Source: CAD feature listing. Evaluate the final solid. Frame: model axes, mm. A direction names the side the tool comes from. Coordinates: 2 decimals unless noted, no trailing zeros. Loops run counter-clockwise (first coordinate to the right, second up) from the corner with the lowest first, then second, coordinate; pieces in that order, holes last.
```python
from build123d import *

# Parameters (mm, degrees)
SKETCH_1_W          = 34
SKETCH_1_H          = 10
EXTRUDE_1_DEPTH     = 2
FILLET_1_R          = 3
SKETCH_2_R          = 1.5
CUT_EXTRUDE_1_DEPTH = 2
EXTRUDE_2_DEPTH     = 11
SKETCH_5_W          = 21
SKETCH_5_H          = 14
EXTRUDE_4_DEPTH     = 2
EXTRUDE_4_TAPER     = 48
SKETCH_6_W          = 15
SKETCH_6_H          = 8
CUT_EXTRUDE_2_DEPTH = 0.3
EXTRUDE_5_DEPTH     = 8


with BuildPart() as part:
    # 草图1 → 凸台-拉伸1 (new body)
    with BuildSketch(Plane.XY):
        Rectangle(SKETCH_1_W, SKETCH_1_H)
    extrude(amount=EXTRUDE_1_DEPTH)

    # 圆角1
    fillet_1_edges = [part.edges().sort_by_distance(p)[0] for p in [
        (-17, 5, 1),
        (17, 5, 1),
        (17, -5, 1),
        (-17, -5, 1),
    ]]
    fillet(fillet_1_edges, radius=FILLET_1_R)

    # 草图2 → 切除-拉伸1 (cut)
    with BuildSketch(Plane.XY.offset(2)):
        with Locations((-14, 0)):
            Circle(SKETCH_2_R)
        with Locations(Location((14, 0, 0), (0, 0, 180))):
            Circle(SKETCH_2_R)
    extrude(amount=-CUT_EXTRUDE_1_DEPTH, mode=Mode.SUBTRACT)

    # 草图3 → 凸台-拉伸2 (add)
    with BuildSketch(Plane.XY.offset(2)):
        with BuildLine():
            Line((12, -5), (-12, -5))
            Line((-12, -5), (-12, -4))
            Line((-12, -4), (-7.5, -4))
            ThreePointArc((-7.5, -4), (-5, -1.5), (-7.5, 1))
            Line((-7.5, 1), (-12, 1))
            Line((-12, 1), (-12, 5))
            Line((-12, 5), (12, 5))
            Line((12, 5), (12, 1))
            Line((12, 1), (7.5, 1))
            ThreePointArc((7.5, 1), (5, -1.5), (7.5, -4))
            Line((7.5, -4), (12, -4))
            Line((12, -4), (12, -5))
        make_face()
    extrude(amount=EXTRUDE_2_DEPTH)

    # 草图5 → 凸台-拉伸4 (add)
    with BuildSketch(Plane.XZ.offset(5)):
        with Locations((0, 6)):
            Rectangle(SKETCH_5_W, SKETCH_5_H)
    extrude(amount=EXTRUDE_4_DEPTH, taper=EXTRUDE_4_TAPER)

    # 草图6 → 切除-拉伸2 (cut)
    with BuildSketch(Plane.XZ.offset(7)):
        with Locations((0, 6)):
            Rectangle(SKETCH_6_W, SKETCH_6_H)
    extrude(amount=-CUT_EXTRUDE_2_DEPTH, mode=Mode.SUBTRACT)

    # 草图8 → 凸台-拉伸5 (add)
    with BuildSketch(Plane.XY.offset(2)):
        with BuildLine():
            Line((7.5, -6.7), (7.5, -7))
            ThreePointArc((7.5, -7), (0.438935642, -8.061882235), (-5.960909355, -11.228616794))
            Line((-5.960909355, -11.228616794), (-7.5, -7))
            Line((-7.5, -7), (-7.5, -6.7))
            Line((-7.5, -6.7), (7.5, -6.7))
        make_face()
    extrude(amount=EXTRUDE_5_DEPTH)


solid = part.part
```
Q1. Section query D-D on y = -3. Return the cut outline in (x, z).
Q2. Section query B-B on x = 13. Return the cut outline in (y, z).
Q3. Material intervals for line 1 along Y through (x, z) = (14, 0.55); line 2 along Z through (x, y) = (-3, -1.5); line 3 along Y through (x, z) = (9.5, 5.25), sorted ascending.
Q4. Section query C-C on y = 4.25. Return the cut outline in (x, z), then the cut area to 3 significant figures.
Q5. First-contact query: pin 1 Ø3 at (y, z) = (-3.5, 11) entering from -X; pin 2 Ø5 at (y, z) = (-6.5, 1) entering from -X; pin 3 Ø5 at (x, y) = (-13.5, -1.5) entering from +Z. Flat tips, straight axial feed; report the tip coordinate or a pass-through.
Q6. Draft query along Y for faces 6 (the cylindrical face through (5, -1.4, 7.4)), 7 (the flat face through (12, 3, 7)), 8 (the flat face through (-10, 1, 7)), 9 (the cylindrical face through (16.1, -4.14, 1.01)). Return one class per face: released by +Y, released by -Y, zero draft, split by the parting line, or undercut.
Q7. Reachability of faces 1 (the flat face through (-12, 3, 7)), 2 (the flat face through (-3, -8, 10)), 3 (the flat face through (-10, -4, 7)), 4 (the flat face through (-3, -8, 2)), 5 (the flat face through (-0.1, -5, -0.5)) from +Z, -Z, +X, -X, +Y, -Y: full face, straight path, thin tool, end or side. Return the list, or none.
Q8. Section query A-A on y = 0. Return the cut outline in (x, z).
Resolved:
1. outline: (-16.83, 0) - (16.83, 0) - (16.83, 2) - (5.5, 2) - (5.5, 13) - (-5.5, 13) - (-5.5, 2) - (-16.83, 2) - close
2. outline: (-5, 0) - (-1.12, 0) - (-1.12, 2) - (-5, 2) - close; (1.12, 0) - (5, 0) - (5, 2) - (1.12, 2) - close
3. line 1: y = -5 to -1.5, 1.5 to 5
3. line 2: z = 0 to 13
3. line 3: y = -5.9 to -4, 1 to 5
4. outline: (-15.98, 0) - (15.98, 0) - (15.98, 2) - (12, 2) - (12, 13) - (-12, 13) - (-12, 2) - (-15.98, 2) - close
4. area: 328 mm2
5. pin 1: stops at x = -12
5. pin 2: stops at x = -16.24
5. pin 3: stops at z = 2
6. face 6: undercut
6. face 7: zero draft
6. face 8: undercut
6. face 9: released by -Y
7. face 1: +Z, -X, +Y, -Y
7. face 2: +Z, +X, -X, -Y
7. face 3: +Z, -X
7. face 4: -Z, +X, -X, -Y
7. face 5: -Z, +X, -X, +Y
8. outline: (-17, 0) - (-15.5, 0) - (-15.5, 2) - (-17, 2) - close; (-12.5, 0) - (12.5, 0) - (12.5, 2) - (5.5, 2) - (5.5, 13) - (-5.5, 13) - (-5.5, 2) - (-12.5, 2) - close; (15.5, 0) - (17, 0) - (17, 2) - (15.5, 2) - close
